Input: part model. Units: mm. Frame: model coordinates. A direction names the side the tool comes from. Round coordinates to 2 decimals unless told otherwise and drop trailing zeros. Loops run counter-clockwise (first coordinate to the right, second up) from the corner with the lowest first, then second, coordinate; pieces in that order, holes last. Notation, with made-up numbers: M 37,28 L 46,28 A13 ccw 46,40 Z; hole C 71.5,24.5 d5. An arc over 180 degrees is marked long. Return JSON: item names as keys, results as strings. Group by question number.
1) Section C-C (z = -3). Output: boundary loops of the cut face in (x, y).
2) Access query for faces 3 (the face through (1, 1, 28)), 4 (the face through (1, 1, 30)), 5 (the face through (1, 1, 62)), 6 (the face through (0, -3.2, 0)). Directions: +Z, -Z, +X, -X, +Y, -Y. A direction counts if a zero-diameter tool reaches every point of the face in a straight line with its end or side. Return the directions, or none.
3) Contact query for flat-ended pins moving along their axis: P1, Ø3, axis at x = -1, y = 0, coming from the -Z side; P2, Ø3, axis at x = 0, y = -0.5, coming from the +Z side; P3, Ø1.2, axis at y = 0, z = -18, coming from the +X side; P4, Ø1.5, axis at x = 3.5, z = 21.5, coming from the -Y side. Output: stop coordinate, or through.
4) Mould query, pull axis Y, two halves, no side actions, for faces 1 (the face through (0, -1, 29)), 2 (the face through (0, 3.3, 0)). Classes: +Y half, -Y half, draft (parallel to the pull), parting line (faces both ways), or undercut.
5) Section A-A (x = 0). Output: boundary loops of the cut face in (y, z).
6) Material intervals for line 1 (Z direction, x = 2.5, y = 1.5); line 2 (Y direction, x = 0, z = 70); line 3 (Y direction, x = 1, z = 6), sorted ascending. Write a range as from..to.
7) Section B-B (z = -18). Output: boundary loops of the cut face in (x, y), plus the area to 3 significant figures.
from build123d import *
from build123d.topology import SkipClean

# Parameters (mm, degrees)
SKETCH2_R               = 4.5
SKETCH2_R_2             = 3
BOSS_EXTRUDE1_DEPTH     = 80
BOSS_EXTRUDE2_START     = 20
BOSS_EXTRUDE2_DEPTH     = 20
CUT_EXTRUDE1_DEPTH      = 81.476704704
CUT_EXTRUDE1_DEPTH_BACK = 81.476704704
SKETCH4_R               = 1
BOSS_EXTRUDE3_START     = 2
SKETCH7_R               = 3
SKETCH7_R_2             = 1
BOSS_EXTRUDE3_DEPTH     = 2
SKETCH10_R              = 3
SKETCH10_R_2            = 1
BOSS_EXTRUDE4_DEPTH     = 2


with BuildPart() as part:
    # Sketch2 → Boss-Extrude1 (new body)
    with BuildSketch(Plane.XY):
        Circle(SKETCH2_R)
        Circle(SKETCH2_R_2, mode=Mode.SUBTRACT)
    extrude(amount=BOSS_EXTRUDE1_DEPTH)

    # Sketch3 → Boss-Extrude2 (add)
    with SkipClean():  # the faces are left unmerged after this step: merging them gives an invalid solid
        with BuildSketch(Plane(origin=(0, 0, 0), x_dir=(-1, 0, 0), z_dir=(0, 0, -1)).offset(BOSS_EXTRUDE2_START)):
            with BuildLine():
                Line((3, 3.354101966), (3, -3.354101966))
                ThreePointArc((3, -3.354101966), (4.5, 0), (3, 3.354101966))
            make_face()
            with BuildLine():
                Line((-3, 3.354101966), (-3, -3.354101966))
                ThreePointArc((-3, -3.354101966), (-4.5, 0), (-3, 3.354101966))
            make_face()
        extrude(amount=-BOSS_EXTRUDE2_DEPTH)

    # Sketch4 → Cut-Extrude1 (cut, two sides: drawn at the far end of the back side and taken through both)
    with SkipClean():  # the faces are left unmerged after this step: merging them gives an invalid solid
        with BuildSketch(Plane.ZY.offset(-3).offset(-CUT_EXTRUDE1_DEPTH_BACK)):
            with Locations((-18, 0)):
                Circle(SKETCH4_R)
        extrude(amount=CUT_EXTRUDE1_DEPTH + CUT_EXTRUDE1_DEPTH_BACK, mode=Mode.SUBTRACT)

    # Sketch7 → Boss-Extrude3 (add)
    with SkipClean():  # the faces are left unmerged after this step: merging them gives an invalid solid
        with BuildSketch(Plane(origin=(0, 0, 30), x_dir=(-1, 0, 0), z_dir=(0, 0, -1)).offset(BOSS_EXTRUDE3_START)):
            Circle(SKETCH7_R)
            Circle(SKETCH7_R_2, mode=Mode.SUBTRACT)
        extrude(amount=-BOSS_EXTRUDE3_DEPTH)

    # Sketch10 → Boss-Extrude4 (add)
    with SkipClean():  # the faces are left unmerged after this step: merging them gives an invalid solid
        with BuildSketch(Plane(origin=(0, 0, 60), x_dir=(-1, 0, 0), z_dir=(0, 0, -1))):
            Circle(SKETCH10_R)
            Circle(SKETCH10_R_2, mode=Mode.SUBTRACT)
        extrude(amount=-BOSS_EXTRUDE4_DEPTH)


solid = part.part
Returned:
{
 "1": {"outline": "M -3,-3.35 L -3,3.35 A4.5 ccw Z; M 3,-3.35 A4.5 ccw 3,3.35 Z"},
 "2": {"face 3": "-Z", "face 4": "none", "face 5": "+Z", "face 6": "-Z, +Y, -Y"},
 "3": {"P1": "stops at z = 28", "P2": "stops at z = 62", "P3": "passes through", "P4": "stops at y = -3.56"},
 "4": {"face 1": "undercut", "face 2": "draft"},
 "5": {"outline": "M -4.5,0 L -3,0 L -3,28 L -1,28 L -1,30 L -3,30 L -3,60 L -1,60 L -1,62 L -3,62 L -3,80 L -4.5,80 Z; M 1,28 L 3,28 L 3,0 L 4.5,0 L 4.5,80 L 3,80 L 3,62 L 1,62 L 1,60 L 3,60 L 3,30 L 1,30 Z"},
 "6": {"line 1": "z = 28..30, 60..62", "line 2": "y = -4.5..-3, 3..4.5", "line 3": "y = -4.39..-2.83, 2.83..4.39"},
 "7": {"outline": "M -4.39,-1 A4.5 ccw -3,-3.35 L -3,-1 Z; M -4.39,1 L -3,1 L -3,3.35 A4.5 ccw Z; M 3,-3.35 A4.5 ccw 4.39,-1 L 3,-1 Z; M 3,1 L 4.39,1 A4.5 ccw 3,3.35 Z", "area": "8.09 mm^2"}
}
